Read the model definition and answer for the solid it produces. Units are mm, in the model's axes. A direction names the side the tool comes from. Round coordinates to 2 decimals unless told otherwise and drop trailing zeros. Order: outer loops, then holes, each group sorted by start corner. A loop starts at its lowest first (then second) coordinate and runs counter-clockwise, first axis right, second up. Notation, with made-up numbers: (3, -19.75) - (61, -19.75) arc R16 ccw to (61, 11.25) - close; hole circle Ø8 at (17.5, -19). An arc over 180 degrees is marked (long way). Put each result on its own line as item: value. Start each with the question number.
Q1. Section B-B on x = 0 is taken. Give the vertices of the cut face in (y, z) (3 decimals), then the cut area to 3 significant figures.
Q2. Section C-C on z = -4.5 is taken. Give the vertices of the cut face in (x, y) (3 decimals), then the cut area to 3 significant figures.
Q3. For a pull along Y with two mould halves and no side action, classify faces 3 (the face through (-0.65, -15.86, -4.85)), 4 (the face through (6.867, 21.804, -3.219)), 5 (the face through (-22, -8, -6.35)) as pulls with the +Y half, pulls with the -Y half, needs draft (parallel to the pull), parting line crosses it, or undercut.
Q4. Section D-D on y = 20 is taken. Give the vertices of the cut face in (x, z).
Q5. Find the intervals of material crossed by line 1 along X through (y, z) = (0, -6) (3 decimals); line 2 along X through (y, z) = (0.5, -7.5); line 3 along Y through (x, z) = (0, -5.5) (3 decimals), in increasing order. Write a range as from..to.
Q6. Section A-A on y = 0 is taken. Give the vertices of the cut face in (x, z) (3 decimals), then the cut area to 3 significant figures.
Q7. Which of the six approach directions +Z, -Z, +X, -X, +Y, -Y give full straight-line access (tool end or side, diameter ignored) to faces 1 (the face through (0, 18.094, -5)), 2 (the face through (-16, 5, 0))?
Q8. Each of these flat-tipped pins is pushed along its axis until it touches: pin 1 Ø5 at (y, z) = (-10.5, -6) entering from -X; pin 2 Ø1.5 at (x, y) = (18, -10) entering from +Z; pin 3 Ø2 at (x, y) = (16.5, -21) entering from +Z; pin 4 Ø2 at (y, z) = (17.5, -7) entering from +X. Where does it stop, or does it pass through?
Autodesk Inventor part; units mm, degrees
ref_plane "YZ Plane" through (0, 0, 0) normal (1, 0, 0) x (0, 1, 0)
ref_plane "XZ Plane" through (0, 0, 0) normal (0, 1, 0) x (-1, 0, 0)
ref_plane "XY Plane" through (0, 0, 0) normal (0, 0, 1) x (1, 0, 0)
sketch "Sketch1" plane through (0, 0, 0) normal (1, 0, 0) x (0, 1, 0)
  line L0 (0, 0) -> (22.86, 0)
  line L1 (22.86, 0) -> (22.86, -6.35)
  line L2 (22.86, -6.35) -> (31.75, -6.35)
  line L3 (31.75, -6.35) -> (31.75, -9.8298)
  line L4 (31.75, -9.8298) -> (0, -9.8298)
  line L5 (0, -9.8298) -> (0, 0)
  dimension "d0" = 22.86
  dimension "d1" = 6.35
  dimension "d2" = 8.89
  dimension "d3" = 3.4798
revolve "Revolution1" add sketch "Sketch1" angle 360 about axis through (0, 0, -9.8298) along (0, 0, 1)
sketch "Sketch2" plane through (0, 0, 0) normal (0, 0, 1) x (1, 0, 0)
  circle A0 centre (0, 0) radius 15.875
  line L0 (-3.175, 15.5543) -> (-3.175, 18.0943)
  line L1 (-3.175, 18.0943) -> (3.175, 18.0943)
  line L2 (3.175, 18.0943) -> (3.175, 15.5543)
  line L3 (0, 0) -> (0, 24.2947)
  point P0 (0, 0)
  point P1 (0, 18.0943)
  dimension "d5" = 31.75
  dimension "d6" = 6.35
  dimension "d7" = 2.54
extrude "Extrusion1" cut sketch "Sketch2" against normal through all
sketch "Sketch3" plane through (0, 0, -6.35) normal (0, 0, 1) x (1, 0, 0)
  point P0 (0, 0)
properties part number "SprocketAdapter"
Findings:
1. outline: (-31.75, -9.83) - (-15.875, -9.83) - (-15.875, 0) - (-22.86, 0) - (-22.86, -6.35) - (-31.75, -6.35) - close; (18.094, -9.83) - (31.75, -9.83) - (31.75, -6.35) - (22.86, -6.35) - (22.86, 0) - (18.094, 0) - close
1. area: 177 mm2
2. outline: circle Ø45.72 at (0, 0); hole (-3.175, 15.554) arc R15.875 ccw (long way) to (3.175, 15.554) - (3.175, 18.094) - (-3.175, 18.094) - close
2. area: 835 mm2
3. face 3: undercut
3. face 4: parting line crosses it
3. face 5: needs draft
4. outline: (-24.66, -9.83) - (24.66, -9.83) - (24.66, -6.35) - (11.07, -6.35) - (11.07, 0) - (-11.07, 0) - (-11.07, -6.35) - (-24.66, -6.35) - close
5. line 1: -22.86..-15.875, 15.875..22.86
5. line 2: -31.75..-15.87, 15.87..31.75
5. line 3: -22.86..-15.875, 18.094..22.86
6. outline: (-31.75, -9.83) - (-15.875, -9.83) - (-15.875, 0) - (-22.86, 0) - (-22.86, -6.35) - (-31.75, -6.35) - close; (15.875, -9.83) - (31.75, -9.83) - (31.75, -6.35) - (22.86, -6.35) - (22.86, 0) - (15.875, 0) - close
6. area: 199 mm2
7. face 1: +Z, -Z
7. face 2: +Z, +X, -X, +Y, -Y
8. pin 1: x = -30.72
8. pin 2: z = 0
8. pin 3: z = -6.35
8. pin 4: x = 27.13
